Answer from the drawing. Dimensions are ordinates in mm from the lowest x, y and z of the part. Coordinates: 2 decimals unless noted, no trailing zeros. Loops run counter-clockwise (first coordinate to the right, second up) from the corner with the lowest first, then second, coordinate; pieces in that order, holes last.
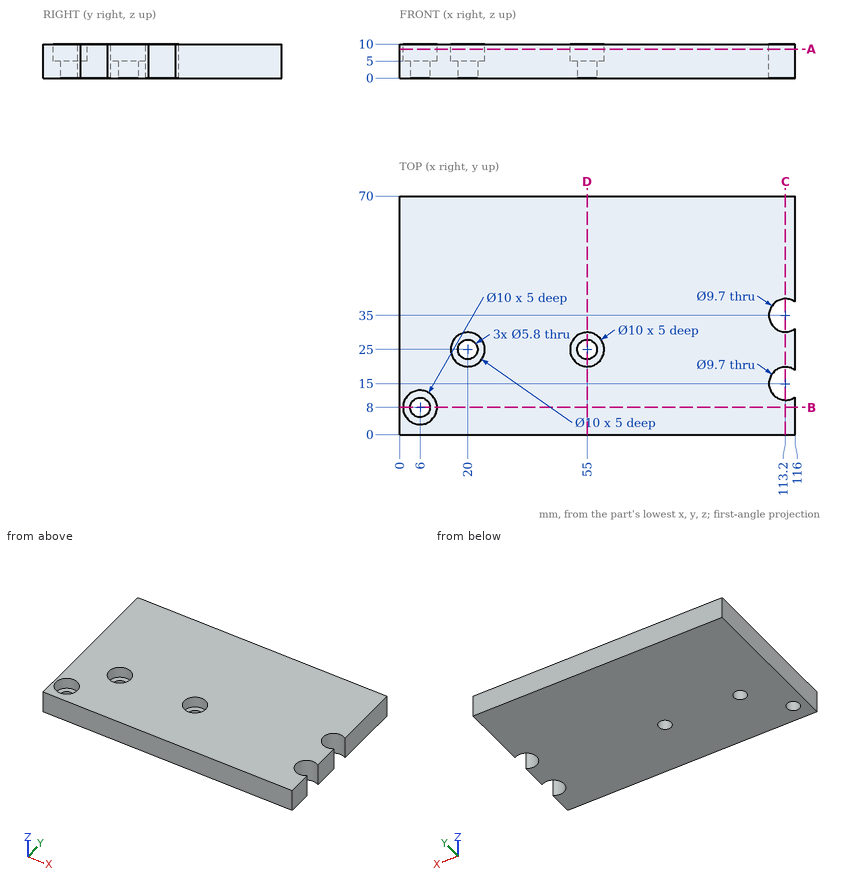
Item 1: A cutting plane is placed at C-C on x = 113.2. Determine the outline of the cut face in (y, z), then the cut area to 3 significant figures.
Numbers:
outline: (0, 0) - (10.15, 0) - (10.15, 10) - (0, 10) - close; (19.85, 0) - (30.15, 0) - (30.15, 10) - (19.85, 10) - close; (39.85, 0) - (70, 0) - (70, 10) - (39.85, 10) - close
area: 506 mm2
Item 2: A cutting plane is placed at D-D on x = 55. Determine the outline of the cut face in (y, z), then the cut area to 3 significant figures.
Numbers:
outline: (0, 0) - (22.1, 0) - (22.1, 5) - (20, 5) - (20, 10) - (0, 10) - close; (27.9, 0) - (70, 0) - (70, 10) - (30, 10) - (30, 5) - (27.9, 5) - close
area: 621 mm2
Item 3: A cutting plane is placed at A-A on z = 8.5. Determine the outline of the cut face in (x, y).
Numbers:
outline: (0, 0) - (116, 0) - (116, 11.04) arc R4.85 cw (long way) to (116, 18.96) - (116, 31.04) arc R4.85 cw (long way) to (116, 38.96) - (116, 70) - (0, 70) - close; hole circle Ø10 at (6, 8); hole circle Ø10 at (20, 25); hole circle Ø10 at (55, 25)
Item 4: Find the intervals of material crossed by line 1 along Y through (x, z) = (113.2, 5.25); line 2 along Y through (x, z) = (6, 8.3); line 3 along Y through (x, z) = (53, 9.5), in increasing order.
Numbers:
line 1: y = 0 to 10.15, 19.85 to 30.15, 39.85 to 70
line 2: y = 0 to 3, 13 to 70
line 3: y = 0 to 20.42, 29.58 to 70
Item 5: Given pin 1 (6 mm diameter, centred on x = 113.2, y = 35, fed in from -Z); pin 2 (5 mm diameter, centred on x = 53.5, y = 25.5, fed in from +Z); pin 3 (1 mm diameter, centred on y = 13.5, z = 2, fed in from +X), each flat-ended and moving along its own axis, determine where each tip first touches the part or whether it passes through.
Numbers:
pin 1: passes through
pin 2: stops at z = 5
pin 3: stops at x = 108.78
Item 6: A cutting plane is placed at B-B on y = 8. Determine the outline of the cut face in (x, z), then the cut area to 3 significant figures.
Numbers:
outline: (0, 0) - (3.1, 0) - (3.1, 5) - (1, 5) - (1, 10) - (0, 10) - close; (8.9, 0) - (116, 0) - (116, 10) - (11, 10) - (11, 5) - (8.9, 5) - close
area: 1,080 mm2
